The model under review builds one solid part; all positions refer to its coordinate system, in mm. A direction names the side the tool comes from. Round coordinates to 2 decimals unless told otherwise and drop trailing zeros. Write each loop counter-clockwise with the first axis right and the second up, starting at its lowest first coordinate (ties: lowest second). Pieces come first, ordered by that corner, then holes. Notation, with made-up numbers: M -25.5,44 L -1.5,44 A29 cw -1.5,65 Z; hole C -34,36 d1. An arc over 180 degrees is marked long. One line per item, written item: value. Start each with the question number.
1) Take a section at A-A, the plane x = 0. Write out the cut boundary in (y, z) (3 decimals), and give its area (3 significant figures).
2) Take a section at C-C, the plane z = -8.5. Write out the cut boundary in (x, y) (3 decimals).
3) Mouldability with a two-part tool opening along Y and no side actions: class faces 4 (the face through (5.5, 0.2, 7.874)), 5 (the face through (-7.095, 5.44, -10.164)), 6 (the face through (-2.77, -4.35, -3.02)) as +Y half, -Y half, draft (parallel to the pull), parting line (faces both ways), or undercut.
4) Tool access review of faces 1 (the face through (4, 4, -14.224)), 2 (the face through (6, -7, -9.576)), 3 (the face through (5, 9, 0)): name each direction out of +Z, -Z, +X, -X, +Y, -Y from which nothing blocks a thin tool from reaching the whole face with its end or side.
5) Take a section at D-D, the plane x = -10. Write out the cut boundary in (y, z).
6) Wall thickness on probe 1 along Y at (x, z) = (0, -7.75) (3 decimals); probe 2 along Z at (x, y) = (2, -10.5); probe 3 along Y at (x, z) = (2, -6.25): over which ranges is each line inside the solid? List them lowest first.
7) For P1, Ø12, axis at y = 6, z = -10.5, coming from the +X side; P2, Ø1.5, axis at y = 3, z = -10.5, coming from the +X side; P3, Ø1, axis at x = 9, z = -11, coming from the +Y side, all flat-tipped, find the tip position at first contact; note any pin that passes through.
from build123d import *

# Parameters (mm, degrees)
F0_R     = 12.7
F1_DEPTH = 7.874
F2_R     = 9.525
F3_DEPTH = 9.5758
F4_R     = 8.9408
F5_DEPTH = 1.1938
F6_R     = 9.5123
F7_DEPTH = 3.4544
F8_SIZE  = 0.762
F10_D    = 10.3124


with BuildPart() as f1:
    # F0 (on Top) → F1 (new body)
    with BuildSketch(Plane.XY):
        Circle(F0_R)
    extrude(amount=F1_DEPTH)

    # F2 (on Top) → F3 (join)
    with BuildSketch(Plane.XY):
        Circle(F2_R)
    extrude(amount=-F3_DEPTH)

    # F4 (on face) → F5 (join)
    with BuildSketch(Plane(origin=(0, 0, -9.5758), x_dir=(1, 0, 0), z_dir=(0, 0, -1))):
        Circle(F4_R)
    extrude(amount=F5_DEPTH)

    # F6 (on face) → F7 (join)
    with BuildSketch(Plane(origin=(0, 0, -10.7696), x_dir=(1, 0, 0), z_dir=(0, 0, -1))):
        Circle(F6_R)
    extrude(amount=F7_DEPTH)

    # F8
    f8_edges = [f1.edges().sort_by_distance(p)[0] for p in [
        (-9.5123, 0, -14.224),
    ]]
    chamfer(f8_edges, length=F8_SIZE)

    # F10 (through all)
    with Locations(Plane(origin=(0, 0, -14.224), x_dir=(1, 0, 0), z_dir=(0, 0, -1))):
        with Locations((0, 0)):
            Hole(F10_D / 2)


solid = f1.part
Checked values:
1. outline: M -12.7,0 L -9.525,0 L -9.525,-9.576 L -8.941,-9.576 L -8.941,-10.77 L -9.512,-10.77 L -9.512,-13.462 L -8.75,-14.224 L -5.156,-14.224 L -5.156,7.874 L -12.7,7.874 Z; M 5.156,-14.224 L 8.75,-14.224 L 9.512,-13.462 L 9.512,-10.77 L 8.941,-10.77 L 8.941,-9.576 L 9.525,-9.576 L 9.525,0 L 12.7,0 L 12.7,7.874 L 5.156,7.874 Z
1. area: 241 mm2
2. outline: C 0,0 d19.05; hole C 0,0 d10.312
3. face 4: draft
3. face 5: parting line
3. face 6: undercut
4. face 1: -Z, +X, -X, +Y, -Y
4. face 2: none
4. face 3: -Z
5. outline: M -7.83,0 L 7.83,0 L 7.83,7.87 L -7.83,7.87 Z
6. probe 1: y = -9.525 to -5.156, 5.156 to 9.525
6. probe 2: z = 0 to 7.87
6. probe 3: y = -9.31 to -4.75, 4.75 to 9.31
7. P1: stops at x = 9.52
7. P2: stops at x = 9.23
7. P3: stops at y = 4.27
